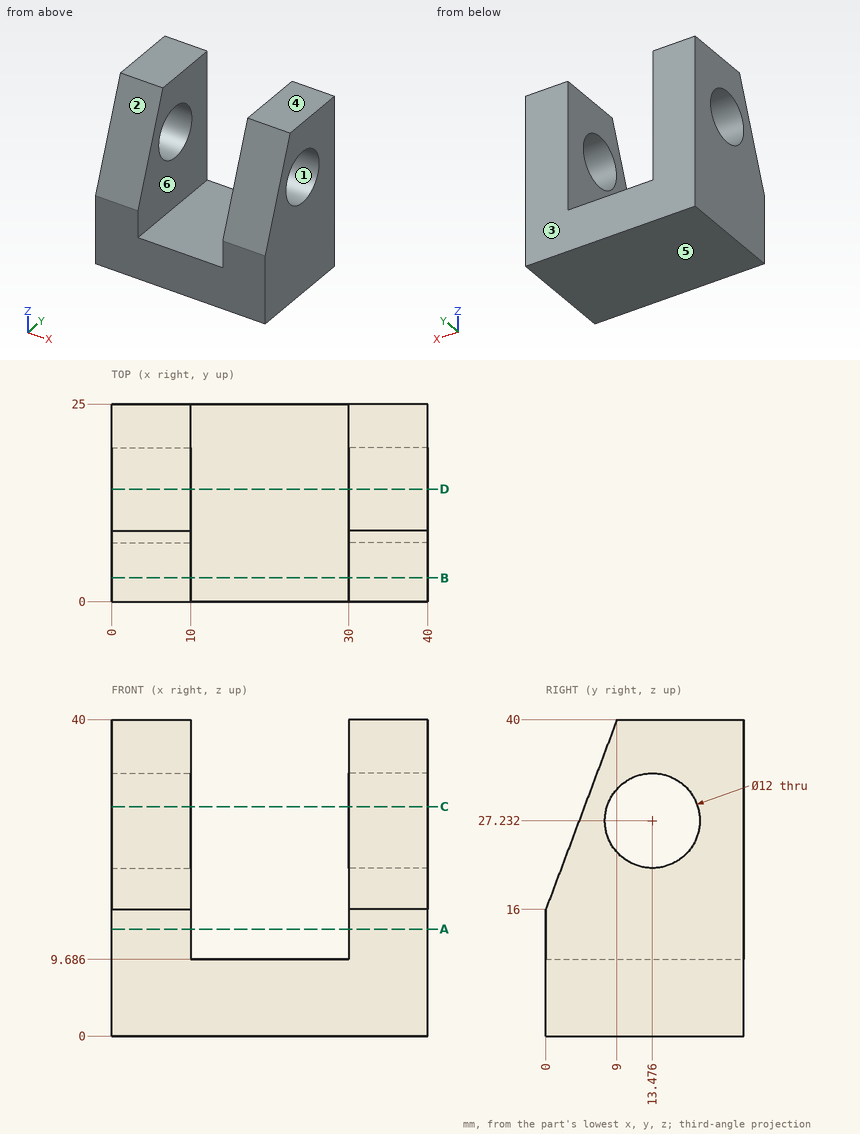
Study the drawing (mm; zero at the part's minimum x, y, z) and answer. A direction names the side the tool comes from. Give positions to 0.01 mm unless a question says otherwise; leave off trailing zeros. Loops run counter-clockwise (first coordinate to the right, second up) from the corner with the lowest first, then second, coordinate; pieces in that order, holes last. Notation, with made-up numbers: (4, -6) -> (51, -6) arc R19 ccw to (51, 11) -> close; hole circle Ø3 at (53.5, 49). An arc over 180 degrees is marked (long way). Write item = value, one per line. Start each with the question number.
(1) The mould has two halves that part along Y. Classify the marked faces 1, 2, 3 and 4: +Y half, -Y half, draft (parallel to the pull), parting line (faces both ways), or undercut.
(2) Find section D-D on y = 14.25. Give the vertices of the cut face in (x, z) (1 decimal).
(3) Find section A-A on z = 13.5. Give the vertices of the cut face in (x, y).
(4) Find section B-B on y = 3. Give the vertices of the cut face in (x, z) (1 decimal).
(5) Find section C-C on z = 29. Give the vertices of the cut face in (x, y) (1 decimal).
(6) Which of the six approach directions +Z, -Z, +X, -X, +Y, -Y give full straight-line access (tool end or side, diameter ignored) to the marked faces 5 and 6?
(7) Find the intervals of material crossed by probe 1 along X at (y, z) = (12.75, 19); probe 2 along Z at (x, y) = (15, 7.75) (1 decimal); probe 3 along Y at (x, z) = (2, 24), in increasing order. Write a range as from..to.
(8) Given pin 1 Ø11 at (y, z) = (13.48, 27.23) entering from +X; pin 2 Ø6 at (x, y) = (21, 13.5) entering from +Z; pin 3 Ø4 at (x, z) = (9.5, 28.5) entering from -Y, each flat-ended and moving along its own axis, determine where each tip first touches the part or whether it passes through.
From the geometry:
q1.face_1 = undercut
q1.face_2 = -Y half
q1.face_3 = +Y half
q1.face_4 = draft
q2.outline = (0, 0) -> (40, 0) -> (40, 21.3) -> (30, 21.3) -> (30, 9.7) -> (10, 9.7) -> (10, 21.3) -> (0, 21.3) -> close; (0, 33.2) -> (10, 33.2) -> (10, 40) -> (0, 40) -> close; (30, 33.2) -> (40, 33.2) -> (40, 40) -> (30, 40) -> close
q3.outline = (0, 0) -> (10, 0) -> (10, 25) -> (0, 25) -> close; (30, 0) -> (40, 0) -> (40, 25) -> (30, 25) -> close
q4.outline = (0, 0) -> (40, 0) -> (40, 24) -> (30, 24) -> (30, 9.7) -> (10, 9.7) -> (10, 24) -> (0, 24) -> close
q5.outline = (0, 4.9) -> (10, 4.9) -> (10, 7.7) -> (0, 7.7) -> close; (0, 19.2) -> (10, 19.2) -> (10, 25) -> (0, 25) -> close; (30, 4.9) -> (40, 4.9) -> (40, 7.7) -> (30, 7.7) -> close; (30, 19.2) -> (40, 19.2) -> (40, 25) -> (30, 25) -> close
q6.face_5 = -Z, +X, -X, +Y, -Y
q6.face_6 = +Z, +Y, -Y
q7.probe_1 = 0..10, 30..40
q7.probe_2 = 0..9.7
q7.probe_3 = 3..8.42, 18.53..25
q8.pin_1 = through
q8.pin_2 = 9.69
q8.pin_3 = 3.94
